Model file for the job. Use its own axes, mm. Give positions to 0.01 mm unless a question says otherwise; leave off trailing zeros. Loops run counter-clockwise (first coordinate to the right, second up) from the corner with the lowest first, then second, coordinate; pieces in that order, holes last. Notation, with made-up numbers: M -2,34.5 L 17,34.5 A14 ccw 17,46.5 Z; hole C 63.25,32.5 d10. An arc over 180 degrees is marked long. Answer in a Markdown table with one row per item.
```python
from build123d import *

# Parameters (mm, degrees)
SKETCH_2_R               = 9.5
SKETCH_2_R_2             = 5
CUT_EXTRUDE_1_DEPTH      = 631.143237685
CUT_EXTRUDE_1_DEPTH_BACK = 631.143237685
SKETCH_3_R               = 5


with BuildPart() as part:
    # По траектории1: sweep along a path in Эскиз1
    with BuildLine(Plane.XY) as sweep_1_path:
        Line((0, 0), (0, -630))
    # Эскиз2 → По траектории1 (sweep)
    with BuildSketch(Plane(origin=(0, 0, 0), x_dir=(1, 0, 0), z_dir=(0, 1, 0))):
        Circle(SKETCH_2_R)
        Circle(SKETCH_2_R_2, mode=Mode.SUBTRACT)
    sweep(path=sweep_1_path.line)

    # Эскиз3 → Вырез-Вытянуть1 (cut, two sides: drawn at the far end of the back side and taken through both)
    with BuildSketch(Plane(origin=(0, 0, 0), x_dir=(0, 0, -1), z_dir=(1, 0, 0)).offset(-CUT_EXTRUDE_1_DEPTH_BACK)):
        with Locations((0, -240)):
            Circle(SKETCH_3_R)
    extrude(amount=CUT_EXTRUDE_1_DEPTH + CUT_EXTRUDE_1_DEPTH_BACK, mode=Mode.SUBTRACT)


solid = part.part
```
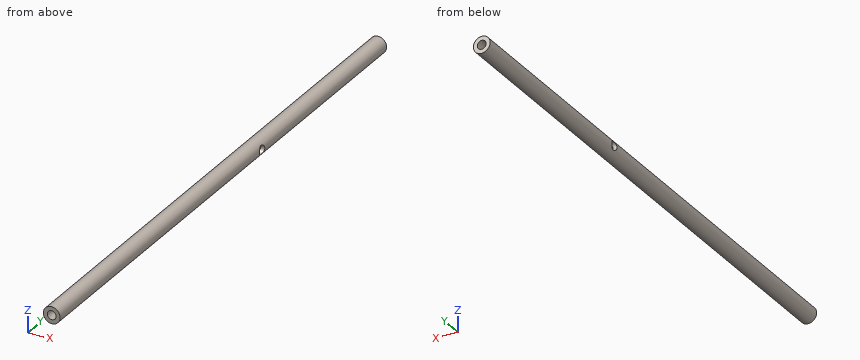
Q1. Probe probe 1 along Y at (x, z) = (7.5, 0); probe 2 along Z at (x, y) = (0, -457.5); probe 3 along X at (y, z) = (-582.5, 0.25). List the from-to ranges inside material, lowest first.
Reported:
| item | result |
|---|---|
| probe 1 | -630 to -245, -235 to 0 |
| probe 2 | -9.5 to -5, 5 to 9.5 |
| probe 3 | -9.5 to -4.99, 4.99 to 9.5 |
Q2. Saw through at B-B (y = -145.5). Give the cut face in (x, z), and give its area (3 significant figures).
Reported:
| item | result |
|---|---|
| outline | C 0,0 d19; hole C 0,0 d10 |
| area | 205 mm² |
Q3. Saw through at A-A (z = 0). Give the cut face in (x, y).
Reported:
| item | result |
|---|---|
| outline | M -9.5,-630 L -5,-630 L -5,-245 L -9.5,-245 Z; M -9.5,-235 L -5,-235 L -5,0 L -9.5,0 Z; M 5,-630 L 9.5,-630 L 9.5,-245 L 5,-245 Z; M 5,-235 L 9.5,-235 L 9.5,0 L 5,0 Z |
Q4. Drop flat-ended pins along their axis: pin 1 (1.5 mm diameter, centred on x = 3.5, z = 0, fed in from -Y); pin 2 (5 mm diameter, centred on y = -78, z = 5, fed in from +X). Give the stop position or say it passes through.
Reported:
| item | result |
|---|---|
| pin 1 | through |
| pin 2 | x = 9.17 |
